Input: part model. Units: mm. Frame: model coordinates. A direction names the side the tool comes from. Coordinates: 2 decimals unless noted, no trailing zeros. Write each loop counter-clockwise with the first axis right and the second up, starting at its lowest first coordinate (ties: lowest second). Pieces come first, ordered by that corner, then holes. Notation, with made-up numbers: (6.25, 36.25) -> (26.25, 36.25) arc R32 cw to (26.25, 62.25) -> close; hole circle Ø11 at (-31.75, 63.25). An arc over 180 degrees is marked (long way). Use one line per item in the form item = value. Start each with the question number.
(1) Cut plane B-B on x = -25. Return the cut outline in (y, z), plus the area to 3 significant figures.
(2) Cut plane D-D on x = 54.5. Return the cut outline in (y, z), plus the area to 3 significant figures.
(3) Cut plane C-C on y = -8.5. Return the cut outline in (x, z), plus the area to 3 significant figures.
(4) Set-up query: faces 1 (the face through (36.118, -1, 54)), 2 (the face through (2, -13, 0)), 3 (the face through (15, -22.86, 22)), 4 (the face through (36.118, -13, 31)). Return all of +Z, -Z, +X, -X, +Y, -Y with unobstructed straight access to the full face (end or side cutting, diameter ignored); none if empty.
(5) Ray query, line 1 along Z through (x, y) = (23.5, -19.75); line 2 along Y through (x, z) = (0, 9.5); line 3 along X through (y, z) = (-1, 67). Return the intervals inside material, ascending.
(6) Pull-direction query (Y, two-part tool) for faces 5 (the face through (15, -2.54, 22)), 6 (the face through (15, 0, 20)), 7 (the face through (36.118, -24, 54)), 8 (the face through (59.363, -13, 38)); classes: released by +Y, released by -Y, zero draft, split by the parting line, or undercut.
(7) First-contact query: pin 1 (22 mm diameter, centred on x = 24, z = 31, fed in from +Y); pin 2 (6 mm diameter, centred on y = -19.5, z = 54, fed in from -X); pin 3 (12 mm diameter, centred on x = -11.5, y = -17, fed in from +Z); pin 4 (3 mm diameter, centred on y = -1.5, z = 59, fed in from -X). Flat tips, straight axial feed; report the tip coordinate or a pass-through.
(8) Cut plane A-A on z = 22. Return the cut outline in (x, y), plus the area to 3 significant figures.
```python
from build123d import *

# Parameters (mm, degrees)
F0_W     = 25.7852114737
F0_H     = 17.4429379404
F1_DEPTH = 25.4
F2_DEPTH = 25.4
F3_T     = 2.54


# Not quite as in the source:
# - a shell that OpenCascade refuses in one call is made with other operations: the cavity is built on its own and cut out


with BuildPart() as f1:
    # F0 (on Front) → F1 (new body)
    with BuildSketch(Plane.XZ):
        Polygon((36.1182577908, 32.5159132481), (-56.2155582011, 32.5159132481), (-56.2155582011, 0), (61.9034692645, 0), (61.9034692645, 32.5159132481), align=None)
        with Locations((49.0108635277, 41.2373822182)):
            Rectangle(F0_W, F0_H)
    extrude(amount=F1_DEPTH)

    # F2 (add): a face of the model
    f2_faces = [f1.faces().sort_by_distance(p)[0] for p in [
        (49.0108635277, -12.7, 49.9588511884),
    ]]
    extrude(f2_faces, amount=F2_DEPTH)

    # F3: shell of thickness 2.54, made by hand


with BuildPart() as f3_core1:
    # F3_t2: copy of F1
    add(f1.part)

    # the walls: a layer under each face that stays
    f3_faces = [f3_core1.faces().sort_by_distance(p)[0] for p in [
        (-10.0486502051, -12.7, 32.5159132481),
        (-36.5290536235, -25.4, 12.5598085314),
        (61.9034692645, -12.7, 37.6794255942),
        (2.8439555317, -12.7, 0),
        (-36.5290536235, 0, 12.5598085314),
        (-56.2155582011, -12.7, 16.257956624),
    ]]
    thicken(f3_faces, amount=-F3_T, mode=Mode.SUBTRACT)


with BuildPart() as f1_1:
    add(f1.part)

    # what is left inside the walls is the cavity
    f3_cavity = [f3_core1.part.solids().sort_by_distance(p)[0] for p in [
        (2.843956, -2.5654, 26.81295),
    ]]
    add(f3_cavity, mode=Mode.SUBTRACT)


solid = f1_1.part
```
Values:
q1.outline = (-25.4, 0) -> (0, 0) -> (0, 32.52) -> (-25.4, 32.52) -> close; hole (-22.86, 2.54) -> (-2.54, 2.54) -> (-2.54, 29.98) -> (-22.86, 29.98) -> close
q1.area = 268 mm2
q2.outline = (-25.4, 0) -> (0, 0) -> (0, 75.36) -> (-2.54, 75.36) -> (-2.54, 2.54) -> (-22.86, 2.54) -> (-22.86, 75.36) -> (-25.4, 75.36) -> close
q2.area = 434 mm2
q3.outline = (-56.22, 0) -> (61.9, 0) -> (61.9, 75.36) -> (59.36, 75.36) -> (59.36, 2.54) -> (-53.68, 2.54) -> (-53.68, 29.98) -> (36.12, 29.98) -> (36.12, 32.52) -> (-56.22, 32.52) -> close
q3.area = 789 mm2
q4.face_1 = +Z, -X, +Y, -Y
q4.face_2 = -Z, +X, -X, +Y, -Y
q4.face_3 = none
q4.face_4 = +Z
q5.line_1 = 0 to 2.54, 29.98 to 32.52
q5.line_2 = -25.4 to -22.86, -2.54 to 0
q5.line_3 = 36.12 to 61.9
q6.face_5 = undercut
q6.face_6 = released by +Y
q6.face_7 = zero draft
q6.face_8 = undercut
q7.pin_1 = 0
q7.pin_2 = 59.36
q7.pin_3 = 32.52
q7.pin_4 = 36.12
q8.outline = (-56.22, -25.4) -> (61.9, -25.4) -> (61.9, 0) -> (-56.22, 0) -> close; hole (-53.68, -22.86) -> (59.36, -22.86) -> (59.36, -2.54) -> (-53.68, -2.54) -> close
q8.area = 703 mm2
